from build123d import *

# Parameters (mm, degrees)
F1_DEPTH      = 50
F2_W          = 30
F2_H          = 40
F3_DEPTH      = 20
F4_W          = 30
F4_H          = 25
F5_DEPTH      = 30
F5_DEPTH_BACK = 25
F6_W          = 20
F6_H          = 20
F7_DEPTH      = 90


with BuildPart() as f1:
    # F0 (on Front) → F1 (new body)
    with BuildSketch(Plane.XZ):
        Polygon((-90, 0), (0, 0), (0, 30), (-30, 30), (-30, 60), (-110, 60), (-110, 40), (-90, 40), align=None)
    extrude(amount=-F1_DEPTH)

    # F2 (on face) → F3 (cut)
    with BuildSketch(Plane(origin=(-110, 0, 0), x_dir=(0, -1, 0), z_dir=(-1, 0, 0))):
        with Locations((-25, 60)):
            Rectangle(F2_W, F2_H)
    extrude(amount=-F3_DEPTH, mode=Mode.SUBTRACT)

    # F4 (on face) → F5 (cut, two sides)
    with BuildSketch(Plane.XY.offset(60)) as f5_sk:
        with Locations((-45, 12.5)):
            Rectangle(F4_W, F4_H)
    extrude(amount=-F5_DEPTH, mode=Mode.SUBTRACT)
    extrude(f5_sk.sketch, amount=-F5_DEPTH_BACK, mode=Mode.SUBTRACT)

    # F6 (on face) → F7 (cut)
    with BuildSketch(Plane.YZ):
        with Locations((25, 0)):
            Rectangle(F6_W, F6_H)
    extrude(amount=-F7_DEPTH, mode=Mode.SUBTRACT)


solid = f1.part
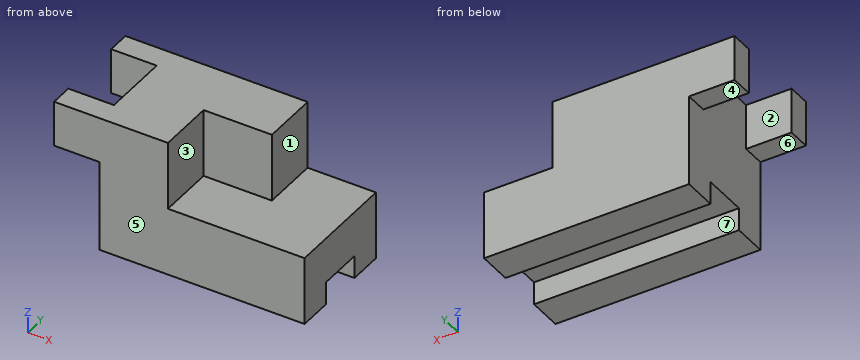
Can you work these out from the model? Positions are in its coordinate system, mm. Face numbers are marked on the shaded views. A direction names the side the tool comes from. Round coordinates to 2 decimals unless told otherwise and drop trailing zeros. Loops run counter-clockwise (first coordinate to the right, second up) from the corner with the lowest first, then second, coordinate; pieces in that order, holes last. Notation, with made-up numbers: (12.25, 2) - (20.25, 2) arc R31 cw to (20.25, 40) - close; hole circle Ø11 at (-9.5, 79). An arc over 180 degrees is marked (long way). Use CSV: the item, a comma, the result in double quotes. Start each with the question number.
1) For pin 1 Ø11 at (x, y) = (-100.5, 6) entering from -Z; pin 2 Ø2 at (y, z) = (21.5, 13.5) entering from -X; pin 3 Ø12.5 at (y, z) = (37, 45.5) entering from +X; pin 4 Ø3 at (x, z) = (-36, 3.5) entering from -Y, each with a flat end and sliding along its axis, tell me the tip position at first contact or that it passes through.
2) If we section it at C-C on z = 50.5: Write out the boundary of the cut face in (x, y), plus the area to 3 significant figures.
3) If we section it at B-B on y = 5: Write out the boundary of the cut face in (x, z).
4) Please list where these lines run through material, in increasing order: probe 1 along Y at (x, z) = (-32.5, 3); probe 2 along X at (y, z) = (12, 10.5); probe 3 along Z at (x, y) = (-20, 48). Write a range as [from, to].
5) For the marked faces 1, 2, 3 and 4, which set-ups out of +Z, -Z, +X, -X, +Y, -Y let a thin tool reach every point of the face, with its end or its side?
6) If we section it at A-A on x = -92: Write out the boundary of the cut face in (y, z), plus the area to 3 significant figures.
7) If we section it at D-D on x = -58: Write out the boundary of the cut face in (y, z).
8) We'd pull the mould along Y, two halves only. Please class the marked faces 5, 6 and 7: released by +Y, released by -Y, zero draft, split by the parting line, or undercut.
Geometry results:
1,pin 1,"stops at z = 40"
1,pin 2,"stops at x = -90"
1,pin 3,"stops at x = -30"
1,pin 4,"stops at y = 0"
2,outline,"(-110, 0) - (-60, 0) - (-60, 25) - (-30, 25) - (-30, 50) - (-110, 50) - (-110, 40) - (-90, 40) - (-90, 10) - (-110, 10) - close"
2,area,"2,650 mm2"
3,outline,"(-110, 40) - (-90, 40) - (-90, 0) - (0, 0) - (0, 30) - (-60, 30) - (-60, 60) - (-110, 60) - close"
4,probe 1,"y = [0, 15], [35, 50]"
4,probe 2,"x = [-90, 0]"
4,probe 3,"z = [0, 30]"
5,face 1,"+Z, +X, +Y, -Y"
5,face 2,"+Z, -Z, -X"
5,face 3,"+Z, +X, -Y"
5,face 4,"-Z, -X, +Y, -Y"
6,outline,"(0, 40) - (10, 40) - (10, 60) - (0, 60) - close; (40, 40) - (50, 40) - (50, 60) - (40, 60) - close"
6,area,"400 mm2"
7,outline,"(0, 0) - (15, 0) - (15, 10) - (35, 10) - (35, 0) - (50, 0) - (50, 60) - (25, 60) - (25, 30) - (0, 30) - close"
8,face 5,"released by -Y"
8,face 6,"zero draft"
8,face 7,"undercut"
